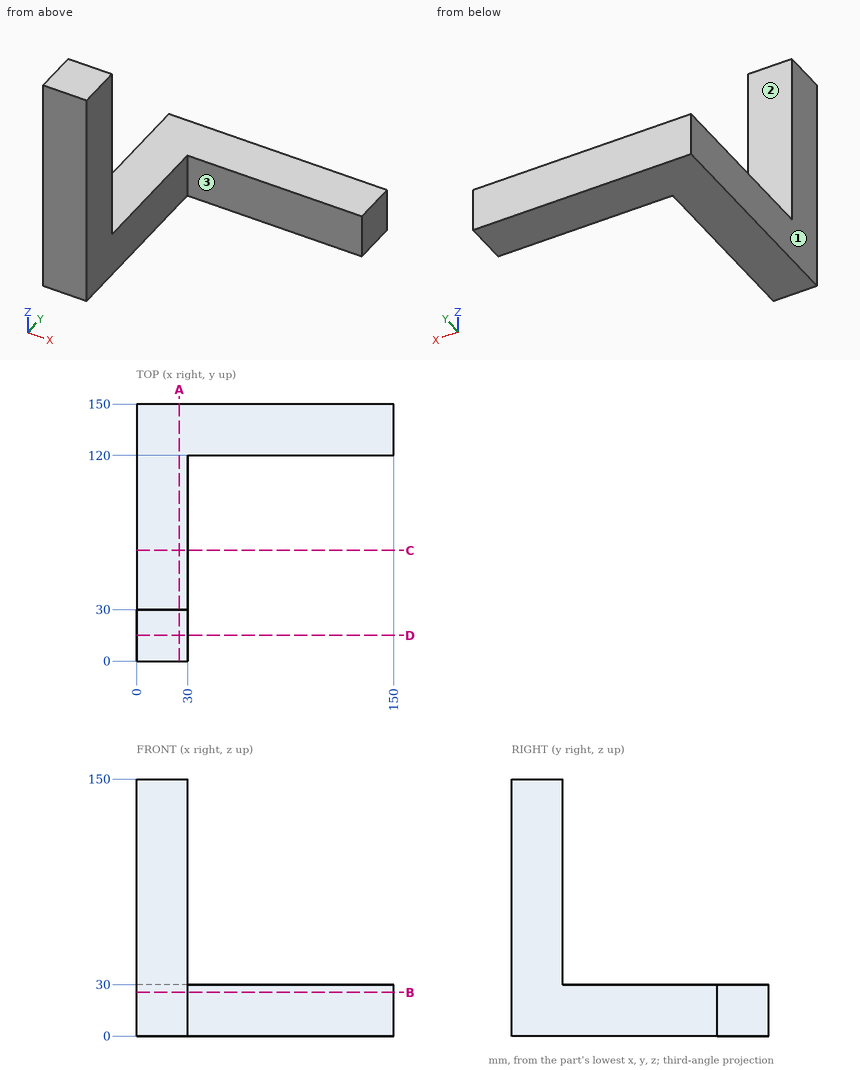
For this review, use the dimensioned drawing (mm, ordinates from the lowest corner) and the shaded views. A direction names the side the tool comes from. Coordinates: 2 decimals unless noted, no trailing zeros. Loops run counter-clockwise (first coordinate to the right, second up) from the corner with the lowest first, then second, coordinate; pieces in that order, holes last. Notation, with made-up numbers: (-2, 4) - (51, 4) arc R13 ccw to (51, 24) - close; hole circle Ø8 at (67.25, 35). An arc over 180 degrees is marked (long way). Use CSV: the item, a comma, the result in double quotes. Start each with the question number.
1) Consider section B-B on z = 25.5. Write out the cut boundary in (x, y).
2) Tool access review of the marked faces 1, 2 and 3: name each direction out of +Z, -Z, +X, -X, +Y, -Y from which nothing blocks a thin tool from reaching the whole face with its end or side.
3) Wall thickness on L1, parallel to Y at x = 131.5, z = 16; L2, parallel to Y at x = 10.5, z = 37.5: over which ranges is each line inside the solid? List them lowest first. Write a range as from..to.
4) Consider section D-D on y = 15. Write out the cut boundary in (x, z), then the cut area to 3 significant figures.
5) For pin 1 Ø3 at (x, z) = (53, 31) entering from -Y; pin 2 Ø9 at (x, z) = (15.5, 79.5) entering from +Y, all flat-tipped, find the tip position at first contact; note any pin that passes through.
6) Consider section A-A on x = 25. Write out the cut boundary in (y, z), then the cut area to 3 significant figures.
7) Consider section C-C on y = 64.5. Write out the cut boundary in (x, z), then the cut area to 3 significant figures.
Geometry says:
1,outline,"(0, 0) - (30, 0) - (30, 120) - (150, 120) - (150, 150) - (0, 150) - close"
2,face 1,"+Z, -Z, -X, +Y, -Y"
2,face 2,"+Z, +X, -X, +Y"
2,face 3,"+Z, -Z, +X, -Y"
3,L1,"120..150"
3,L2,"0..30"
4,outline,"(0, 0) - (30, 0) - (30, 150) - (0, 150) - close"
4,area,"4,500 mm^2"
5,pin 1,"y = 120"
5,pin 2,"y = 30"
6,outline,"(0, 0) - (150, 0) - (150, 30) - (30, 30) - (30, 150) - (0, 150) - close"
6,area,"8,100 mm^2"
7,outline,"(0, 0) - (30, 0) - (30, 30) - (0, 30) - close"
7,area,"900 mm^2"
